```python
from build123d import *

# Parameters (mm, degrees)
F0_W     = 228
F0_H     = 46
F1_DEPTH = 715
F2_T     = -3
F3_R     = 5
F3_R_2   = 5.279175
F4_DEPTH = 3


with BuildPart() as f1:
    # F0 (on Right) → F1 (new body)
    with BuildSketch(Plane.YZ):
        with Locations((65.187312, -3.430253)):
            Rectangle(F0_W, F0_H)
    extrude(amount=F1_DEPTH)

    # F2
    f2_openings = [f1.faces().sort_by_distance(p)[0] for p in [
        (357.5, 65.187312, -26.430253),
    ]]
    offset(amount=F2_T, openings=f2_openings)

    # F3 (on face) → F4 (cut)
    with BuildSketch(Plane.XZ.offset(48.812688)):
        with Locations((659, 0.569747)):
            Circle(F3_R)
        with Locations((272, 0.569747)):
            Circle(F3_R_2)
    extrude(amount=-F4_DEPTH, mode=Mode.SUBTRACT)


solid = f1.part
```
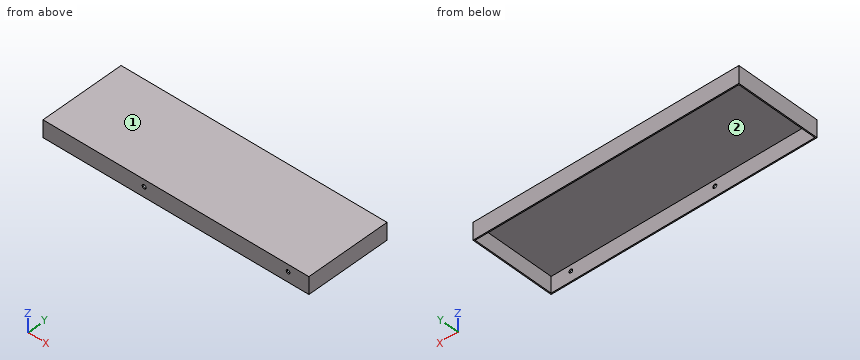
Design review of the part built by this model. Coordinates are the model's own, in mm. Face numbers are marked on the shaded views. Coordinates: 2 decimals unless noted, no trailing zeros. Order: outer loops, then holes, each group sorted by start corner. A loop starts at its lowest first (then second) coordinate and runs counter-clockwise, first axis right, second up. Notation, with made-up numbers: M 13,86 L 25,86 A21 ccw 25,105 Z; hole C 73.5,63.5 d3. An arc over 180 degrees is marked long. Answer as a JSON object with one key per item and string values. Group by question number.
1) Add section C-C, the plane y = 148. Write out the cut boundary in (x, z).
2) Add section A-A, the plane x = 552.5. Write out the cut boundary in (y, z), then the cut area to 3 significant figures.
3) Add section B-B, the plane z = -14.5. Write out the cut boundary in (x, y), then the cut area to 3 significant figures.
4) Wall thickness on L1, parallel to X at y = -18, z = -3.5; L2, parallel to Y at x = 534, z = -17.5; L3, parallel to Z at x = 659, y = -46: over which ranges is each line inside the solid? List them lowest first.
5) For pin 1 (6 mm diameter, centred on x = 299, y = 112, fed in from -Z), flat-tipped, find the tip position at first contact; note if it passes through.
6) Mouldability with a two-part tool opening along Y and no side actions: class the marked faces 1 and 2 as pulls with the +Y half, pulls with the -Y half, needs draft (parallel to the pull), parting line crosses it, or undercut.
Computed values:
{
 "1": {"outline": "M 0,-26.43 L 3,-26.43 L 3,16.57 L 712,16.57 L 712,-26.43 L 715,-26.43 L 715,19.57 L 0,19.57 Z"},
 "2": {"outline": "M -48.81,-26.43 L -45.81,-26.43 L -45.81,16.57 L 176.19,16.57 L 176.19,-26.43 L 179.19,-26.43 L 179.19,19.57 L -48.81,19.57 Z", "area": "942 mm^2"},
 "3": {"outline": "M 0,-48.81 L 715,-48.81 L 715,179.19 L 0,179.19 Z; hole M 3,-45.81 L 712,-45.81 L 712,176.19 L 3,176.19 Z", "area": "5,620 mm^2"},
 "4": {"L1": "x = 0 to 3, 712 to 715", "L2": "y = -48.81 to -45.81, 176.19 to 179.19", "L3": "z = -26.43 to -4.43, 5.57 to 19.57"},
 "5": {"pin 1": "stops at z = 16.57"},
 "6": {"face 1": "needs draft", "face 2": "undercut"}
}
